```python
from build123d import *

# Parameters (mm, degrees)
F0_W     = 42
F0_H     = 22
F1_DEPTH = 5
F2_W     = 42
F2_H     = 22
F3_DEPTH = 2
F4_W     = 42
F4_H     = 22
F4_W_2   = 40.2
F4_H_2   = 20.2
F5_DEPTH = 2
F6_R     = 5


with BuildPart() as f1:
    # F0 (on Top) → F1 (new body)
    with BuildSketch(Plane.XY):
        with Locations((2.120368, 5.306732)):
            Rectangle(F0_W, F0_H)
        with BuildLine():
            ThreePointArc((0, 0), (-17.379632, 5.306732), (0, 10.613464))
            Line((0, 10.613464), (4.240737, 10.613464))
            ThreePointArc((4.240737, 10.613464), (14.89467, 14.392614), (21.620368, 5.306732))
            ThreePointArc((21.620368, 5.306732), (14.89467, -3.77915), (4.240737, 0))
            Line((4.240737, 0), (0, 0))
        make_face(mode=Mode.SUBTRACT)
    extrude(amount=F1_DEPTH)

    # F2 (on face) → F3 (join)
    with BuildSketch(Plane(origin=(0, 0, 0), x_dir=(1, 0, 0), z_dir=(0, 0, -1))):
        with Locations((2.120368, -5.306732)):
            Rectangle(F2_W, F2_H)
    extrude(amount=F3_DEPTH)

    # F4 (on face) → F5 (cut)
    with BuildSketch(Plane.XY.offset(5)):
        with Locations((2.120368, 5.306732)):
            Rectangle(F4_W, F4_H)
        with Locations((2.120368, 5.306732)):
            Rectangle(F4_W_2, F4_H_2, mode=Mode.SUBTRACT)
    extrude(amount=-F5_DEPTH, mode=Mode.SUBTRACT)

    # F6
    f6_edges = [f1.edges().sort_by_distance(p)[0] for p in [
        (-18.879632, 16.306732, 0.5),
        (-18.879632, -5.693268, 0.5),
        (23.120368, -5.693268, 0.5),
        (23.120368, 16.306732, 0.5),
        (22.220368, 15.406732, 4),
        (-17.979632, -4.793268, 4),
        (22.220368, -4.793268, 4),
        (-17.979632, 15.406732, 4),
    ]]
    fillet(f6_edges, radius=F6_R)


solid = f1.part
```
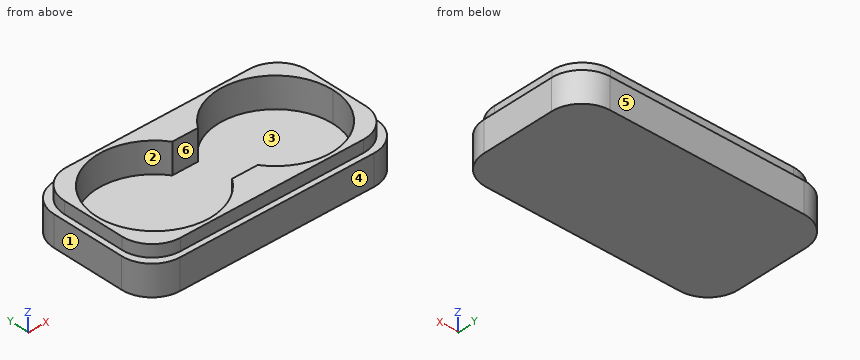
Geometry: final body of the model. Coordinates: model frame, mm. Face numbers are marked on the shaded views. A direction names the side the tool comes from. Round coordinates to 2 decimals unless told otherwise and drop trailing zeros. Write each loop counter-clockwise with the first axis right and the second up, starting at its lowest first coordinate (ties: lowest second). Pieces come first, ordered by that corner, then holes.
Item 1: Section query B-B (x = -12). Return loops of the section in (y, z), plus the area to 3 significant figures.
Item 2: Section query D-D (y = 8). Return loops of the section in (x, z), plus the area to 3 significant figures.
Item 3: Material intervals for L1, parallel to Y at x = 2, z = 2.5; L2, parallel to X at y = 12.25, z = 0.5; L3, parallel to Y at x = -8, z = 1.5, sorted ascending.
Item 4: Pin query (flat end, axial travel): P1, Ø4, axis at x = 10, y = 11, coming from the +Z side; P2, Ø1.6, axis at y = 3, z = 4, coming from the -X side. Return the tip coordinate at first contact, or that it passes through.
Item 5: Mould query, pull axis Y, two halves, no side actions, for the marked faces 3, 4, 5 and 6. Classes: +Y half, -Y half, draft (parallel to the pull), parting line (faces both ways), or undercut.
Item 6: Section query A-A (z = 1.5). Return loops of the section in (x, y).
Item 7: Section query C-C (z = -0.5). Return loops of the section in (x, y).
Item 8: Set-up query: the marked faces 1 and 2. Return all of +Z, -Z, +X, -X, +Y, -Y with unobstructed straight access to the full face (end or side cutting, diameter ignored); none if empty.
Completed:
1. outline: (-5.69, -2) - (16.31, -2) - (16.31, 3) - (15.41, 3) - (15.41, 5) - (13.87, 5) - (13.87, 0) - (-3.25, 0) - (-3.25, 5) - (-4.79, 5) - (-4.79, 3) - (-5.69, 3) - close
1. area: 64.8 mm2
2. outline: (-18.88, -2) - (23.12, -2) - (23.12, 3) - (22.22, 3) - (22.22, 5) - (21.23, 5) - (21.23, 0) - (-16.99, 0) - (-16.99, 5) - (-17.98, 5) - (-17.98, 3) - (-18.88, 3) - close
2. area: 99.3 mm2
3. L1: y = -5.69 to 0, 10.61 to 16.31
3. L2: x = -18.79 to -14.36, -1.4 to 5.64, 18.6 to 23.03
3. L3: y = -5.69 to -4.19, 14.81 to 16.31
4. P1: stops at z = 0
4. P2: stops at x = -17.98
5. face 3: undercut
5. face 4: -Y half
5. face 5: +Y half
5. face 6: undercut
6. outline: (-18.88, -0.69) arc R5 ccw to (-13.88, -5.69) - (18.12, -5.69) arc R5 ccw to (23.12, -0.69) - (23.12, 11.31) arc R5 ccw to (18.12, 16.31) - (-13.88, 16.31) arc R5 ccw to (-18.88, 11.31) - close; hole (0, 0) - (4.24, 0) arc R9.5 ccw to (21.62, 5.31) arc R9.5 ccw to (4.24, 10.61) - (0, 10.61) arc R9.5 ccw (long way) to start
7. outline: (-18.88, -0.69) arc R5 ccw to (-13.88, -5.69) - (18.12, -5.69) arc R5 ccw to (23.12, -0.69) - (23.12, 11.31) arc R5 ccw to (18.12, 16.31) - (-13.88, 16.31) arc R5 ccw to (-18.88, 11.31) - close
8. face 1: +Z, -Z, -X, +Y, -Y
8. face 2: +Z
